from build123d import *

# Parameters (mm, degrees)
F3_DEPTH = 50
F4_DEPTH = 50
F5_DEPTH = 50


with BuildPart() as f3:
    # F0 (on Top) → F3 (new body, symmetric)
    with BuildSketch(Plane.XY):
        Polygon((50, -36.094326), (30, -36.094326), (-29, -36.094326), (-29, -17.455937), (30, -17.455937), (46.441259, -17.455937), (46.441259, 42.544063), (30, 42.544063), (-50, 42.544063), (-50, 12.319882), (15.221381, 12.319882), (15.221381, 0), (-50, 0), (-50, -50), (30, -50), (50, -50), align=None)
    extrude(amount=F3_DEPTH, both=True)

    # F1 (on Front) → F4 (intersect, symmetric)
    with BuildSketch(Plane.XZ):
        with BuildLine():
            Line((0.401398, 47.279804), (-47.496608, 47.684579))
            Line((-47.496608, 47.684579), (-47.496608, -47.940426))
            Line((-47.496608, -47.940426), (0, -47.940426))
            ThreePointArc((0, -47.940426), (33.587572, -34.027999), (47.5, -0.440426))
            Line((47.5, -0.440426), (47.5, -0.2185))
            ThreePointArc((47.5, -0.2185), (33.729189, 33.226855), (0.401398, 47.279804))
        make_face()
        with BuildLine():
            Line((-16.25, -16.25), (-16.25, 16.25))
            Line((-16.25, 16.25), (0, 16.25))
            ThreePointArc((0, 16.25), (11.490485, 11.490485), (16.25, 0))
            ThreePointArc((16.25, 0), (11.490485, -11.490485), (0, -16.25))
            Line((0, -16.25), (-16.25, -16.25))
        make_face(mode=Mode.SUBTRACT)
    extrude(amount=F4_DEPTH, both=True, mode=Mode.INTERSECT)

    # F2 (on Right) → F5 (intersect, symmetric)
    with BuildSketch(Plane.YZ):
        Polygon((14.925366, 50.447736), (-5.373133, -8.95522), (-29.727991, 48.903065), (-55.721365, 48.903065), (-55.721365, -51.030165), (-25.97014, -50.642264), (-25.97014, 6.567161), (-5.373133, -39.960397), (15.223874, 6.567161), (15.223874, -50.642264), (55.721365, -50.114252), (55.721365, 50.447736), align=None)
    extrude(amount=F5_DEPTH, both=True, mode=Mode.INTERSECT)


solid = f3.part
CAD build for the part. Positions are in the model's coordinates, mm. A direction names the side the tool comes from. Round coordinates to 2 decimals unless told otherwise and drop trailing zeros. Order: outer loops, then holes, each group sorted by start corner. A loop starts at its lowest first (then second) coordinate and runs counter-clockwise, first axis right, second up. Notation, with made-up numbers: M 29,54 L 50,54 A26 cw 50,79 Z; hole C -14,62 d3. An arc over 180 degrees is marked long. Use one line per item in the form item = value.
Q1. Saw through at B-B on y = 26. Give the cut face in (x, z).
Recorded:
outline = M -47.5,-47.94 L 0,-47.94 A47.5 ccw 46.44,-10.41 L 46.44,9.75 A47.5 ccw 0.4,47.28 L -47.5,47.68 Z; hole M -16.25,-16.25 L 0,-16.25 A16.25 ccw 16.25,0 A16.25 ccw 0,16.25 L -16.25,16.25 Z
Q2. Two-plate mould, pull along Y, no slides. Class faces 1 (the flat face through (-22, -50, 1)), 2 (the flat face through (-24, 29, -47.94)), 3 (the flat face through (-10.31, -17.13, 18.97)), 4 (the flat face through (-21, 42.544, 1)): +Y half, -Y half, draft (parallel to the pull), parting line (faces both ways), or undercut.
Recorded:
face_1 = -Y half
face_2 = draft
face_3 = undercut
face_4 = +Y half
Q3. Which spindle directions (+Z, -Z, +X, -X, +Y, -Y) get a long thin tool onto all of the face, cutting with end or side? Do faces 5 (the flat face through (-8, -43, -16.25)), 6 (the flat face through (18, -36.094, 0)), 7 (the flat face through (-23, 0, -14)), 8 (the flat face through (-38, -25.97, -21)). Say none if no direction does.
Recorded:
face_5 = +Y, -Y
face_6 = +Z, -Z, +X
face_7 = +Z, -Z, -X
face_8 = -Z, +X, -X
Q4. Flat gauge pins, fed straight in: P1, Ø4, axis at x = -6, y = -44, coming from the +Z side; P2, Ø5, axis at x = -4.5, y = 26.5, coming from the +Z side; P3, Ø5, axis at y = 3, z = -13, coming from the -X side. Where does each tip first touch, or does it go through?
Recorded:
P1 = 47.35
P2 = 47.34
P3 = 15.22
Q5. Probe L1, parallel to X at y = -14, z = 1; L2, parallel to Y at x = -18.5, z = 9; L3, parallel to Y at x = 19.5, z = -37.5. List the from-to ranges inside material, lowest first.
Recorded:
L1 = -47.5 to -16.25, 16.22 to 46.44
L2 = -50 to -36.09, -17.46 to -12.93, 12.32 to 42.54
L3 = -50 to -36.09, -6.46 to -4.28, 15.22 to 42.54
Q6. Saw through at D-D on x = -3.5. Give the cut face in (y, z), then the cut area to 3 significant figures.
Recorded:
outline = M -50,-47.94 L -36.09,-47.94 L -36.09,-16.25 L -50,-16.25 Z; M -50,16.25 L -36.09,16.25 L -36.09,47.31 L -50,47.31 Z; M -17.46,16.25 L -15.98,16.25 L -17.46,19.75 Z; M -15.87,-16.25 L -5.37,-39.96 L 0,-27.82 L 0,-16.25 Z; M 12.32,16.25 L 42.54,16.25 L 42.54,47.31 L 13.85,47.31 L 12.32,42.82 Z; M 15.22,-47.94 L 42.54,-47.94 L 42.54,-16.25 L 15.22,-16.25 Z
area = 2,900 mm^2
Q7. Saw through at A-A on z = 32. Give the cut face in (x, y).
Recorded:
outline = M -47.5,-50 L 34.9,-50 L 34.9,-36.09 L -29,-36.09 L -29,-22.61 L -47.5,-22.61 Z; M -47.5,12.32 L 15.22,12.32 L 15.22,8.62 L 34.9,8.62 L 34.9,42.54 L -47.5,42.54 Z
Q8. Saw through at C-C on x = 22. Give the cut face in (y, z).
Recorded:
outline = M -50,-42.54 L -36.09,-42.54 L -36.09,41.88 L -50,41.88 Z; M -17.46,-12.67 L -5.37,-39.96 L 15.22,6.57 L 15.22,-42.54 L 42.54,-42.54 L 42.54,41.88 L 12,41.88 L -5.37,-8.96 L -17.46,19.75 Z
